Print and shaded views of the part. All mm, measured from the part's lowest x, y and z. Coordinates: 2 decimals unless noted, no trailing zeros. Order: outer loops, then holes, each group sorted by start corner. A loop starts at its lowest first (then second) coordinate and runs counter-clockwise, first axis right, second up. Notation, with made-up numbers: (-28, -36.5) -> (-23, -36.5) arc R31 cw to (-23, 1.5) -> close; hole circle Ø4 at (67.5, -11). An arc over 180 degrees is marked (long way). Return JSON: item names as keys, results as strings. Group by question number.
1) Cut at B-B (z = 66.04). Write the cut outline in (x, y), and give its area (3 significant figures).
2) Cut at A-A (x = 66.04). Write the cut outline in (y, z), and give its area (3 significant figures).
3) Cut at D-D (z = 8). Write the cut outline in (x, y), and give its area (3 significant figures).
4) Flat gauge pins, fed straight in: pin 1 (7.5 mm diameter, centred on x = 21.83, z = 81.92, fed in from -Y); pin 2 (5.5 mm diameter, centred on x = 110.25, z = 50.17, fed in from +Y); pin 3 (5 mm diameter, centred on y = 6.5, z = 81.5, fed in from -X); pin 4 (5 mm diameter, centred on x = 36, y = 10, fed in from +Z). Where does each tip first touch, or does it go through?
5) Probe line 1 (X direction, y = 3.5, z = 66.04); line 2 (Z direction, x = 19.5, y = 9.75) (1 decimal); line 3 (X direction, y = 11.25, z = 112). List the from-to ranges inside material, lowest first.
6) Cut at C-C (y = 4). State how many separate pieces and enclosed holes the cut face has, and give its area (3 significant figures).
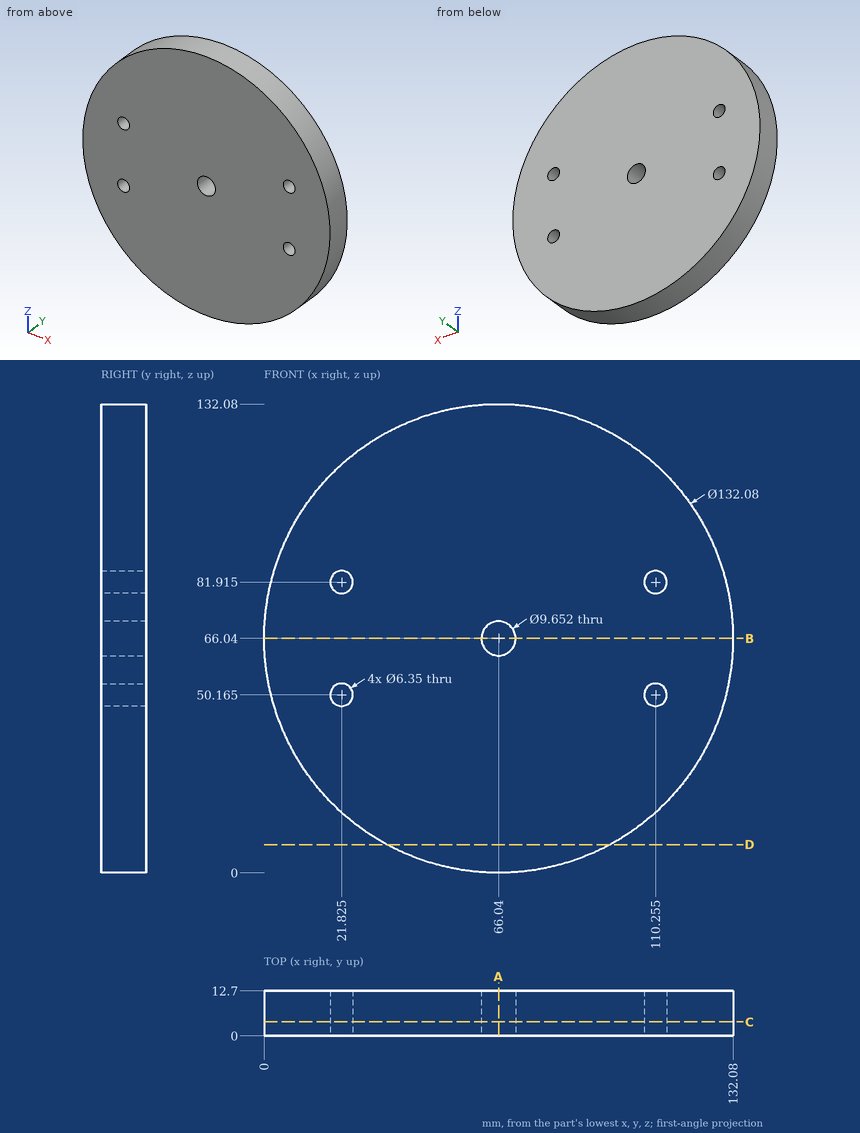
Answers below:
{
 "1": {"outline": "(0, 0) -> (61.21, 0) -> (61.21, 12.7) -> (0, 12.7) -> close; (70.87, 0) -> (132.08, 0) -> (132.08, 12.7) -> (70.87, 12.7) -> close", "area": "1,550 mm^2"},
 "2": {"outline": "(0, 0) -> (12.7, 0) -> (12.7, 61.21) -> (0, 61.21) -> close; (0, 70.87) -> (12.7, 70.87) -> (12.7, 132.08) -> (0, 132.08) -> close", "area": "1,550 mm^2"},
 "3": {"outline": "(34.53, 0) -> (97.55, 0) -> (97.55, 12.7) -> (34.53, 12.7) -> close", "area": "800 mm^2"},
 "4": {"pin 1": "stops at y = 0", "pin 2": "passes through", "pin 3": "stops at x = 1.28", "pin 4": "stops at z = 126.06"},
 "5": {"line 1": "x = 0 to 61.21, 70.87 to 132.08", "line 2": "z = 19.2 to 48, 52.3 to 79.8, 84.1 to 112.9", "line 3": "x = 18.62 to 113.46"},
 "6": {"separate pieces": "1", "enclosed holes": "5", "area": "13,500 mm^2"}
}
